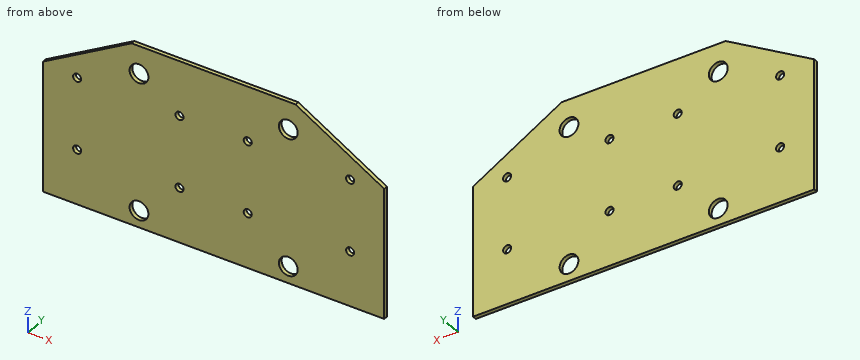
Autodesk Inventor part; units mm, degrees
ref_plane "YZ Plane" through (0, 0, 0) normal (1, 0, 0) x (0, 1, 0)
ref_plane "XZ Plane" through (0, 0, 0) normal (0, 1, 0) x (-1, 0, 0)
ref_plane "XY Plane" through (0, 0, 0) normal (0, 0, 1) x (1, 0, 0)
sketch "Sketch1" plane through (0, 0, 0) normal (0, 1, 0) x (-1, 0, 0)
  line L0 (-63.5, 33.655) -> (63.5, 33.655)
  line L1 (63.5, 33.655) -> (63.5, -33.655)
  line L2 (63.5, -33.655) -> (-63.5, -33.655)
  line L3 (-63.5, -33.655) -> (-63.5, 33.655)
  line L4 (-63.5, 33.655) -> (63.5, -33.655) construction
  line L5 (63.5, 33.655) -> (-63.5, -33.655) construction
  point P0 (0, 0)
  dimension "d0" = 127
  dimension "d1" = 67.31
extrude "Extrusion1" add sketch "Sketch1" along normal mid plane 1.524
sketch "Sketch2" plane through (0, 0.762, 0) normal (0, 1, 0) x (1, 0, 0)
  line L0 (63.5, 33.655) -> (-63.5, 33.655)
  line L1 (-63.5, -33.655) -> (63.5, -33.655)
  line L2 (-63.5, 33.655) -> (-63.5, -33.655)
  line L3 (63.5, -33.655) -> (63.5, 33.655)
  point P0 (0, 0)
  point P1 (-50.8, 13.335)
  point P2 (-12.7, 13.335)
  point P3 (12.7, 13.335)
  point P4 (50.8, 13.335)
  point P5 (50.8, -13.335)
  point P6 (12.7, -13.335)
  point P7 (-12.7, -13.335)
  point P8 (-50.8, -13.335)
  point P9 (-50.8, -33.655)
  point P10 (50.8, -33.655)
  point P11 (-63.5, -20.955)
  point P12 (63.5, -20.955)
  dimension "d5" = 20.32
  dimension "d6" = 20.32
  dimension "d7" = 12.7
  dimension "d8" = 50.8
  dimension "d9" = 12.7
  dimension "d10" = 50.8
hole "Hole1" at (-50.8, 0.762, -13.335) at (-12.7, 0.762, -13.335) at (12.7, 0.762, -13.335) at (50.8, 0.762, -13.335) at (50.8, 0.762, 13.335) at (12.7, 0.762, 13.335) at (-12.7, 0.762, 13.335) at (-50.8, 0.762, 13.335) direction (0, -1, 0) diameter 3 depth 25.4 tip angle 118
chamfer "Chamfer1" distance 19.05 angle 60 1 edges at (-63.5, 0, 33.655) measured on face at (-63.5, -0.254, 11.2183)
sketch "Sketch4" plane through (0, -0.762, 0) normal (0, -1, 0) x (1, 0, 0)
  circle A0 centre (-27.7751, -27.4042) radius 1.7018
  circle A1 centre (-27.7751, 23.3958) radius 1.7018
  circle A2 centre (27.7749, 23.3958) radius 1.7018
  circle A3 centre (27.7749, -27.4042) radius 1.7018
  point P0 (0, 0)
hole "Hole3" at (-27.7751, -0.762, -27.4042) at (-27.7751, -0.762, 23.3958) at (27.7749, -0.762, 23.3958) at (27.7749, -0.762, -27.4042) direction (0, 1, 0) diameter 7 end through all
chamfer "Chamfer2" distance 19.05 angle 60 1 edges at (63.5, 0, 33.655) measured on face at (63.5, 0.254, 11.2183)
properties part number "DPLX_P023 Spark Gap Shielding Bottom" material "Polyethylene, High Density"
Can you work these out from the model? Positions are in its coordinate system, mm. Give positions to 0.01 mm unless a question says otherwise; leave off trailing zeros. Order: outer loops, then holes, each group sorted by start corner. A loop starts at its lowest first (then second) coordinate and runs counter-clockwise, first axis right, second up. Notation, with made-up numbers: M 39,3.25 L 98,3.25 A17 cw 98,8.25 Z; hole C 1,4.25 d3. An arc over 180 degrees is marked long. One line per item, written item: value.
Item 1: Please list where these lines run through material, in increasing order: line 1 (Z direction, x = -12.7, y = 0.2) (3 decimals); line 2 (X direction, y = 0.5, z = -24.5); line 3 (Z direction, x = -29.5, y = 0.65) (3 decimals).
Verdict:
line 1: -33.655 to -14.835, -11.835 to 11.835, 14.835 to 33.655
line 2: -63.5 to -29.73, -25.82 to 25.82, 29.73 to 63.5
line 3: -33.655 to -30.45, -24.359 to 20.35, 26.441 to 33.655
Item 2: If we section it at A-A on x = -12.7: Write out the boundary of the cut face in (y, z) (3 decimals), and give its area (3 significant figures).
Verdict:
outline: M -0.762,-33.655 L 0.762,-33.655 L 0.762,-14.835 L -0.762,-14.835 Z; M -0.762,-11.835 L 0.762,-11.835 L 0.762,11.835 L -0.762,11.835 Z; M -0.762,14.835 L 0.762,14.835 L 0.762,33.655 L -0.762,33.655 Z
area: 93.4 mm2
Item 3: If we section it at D-D on x = -32.5: Write out the boundary of the cut face in (y, z) (3 decimals).
Verdict:
outline: M -0.762,-33.655 L 0.762,-33.655 L 0.762,32.503 L -0.762,32.503 Z
Item 4: If we section it at B-B on y = 0.45: State how many separate pieces and enclosed holes the cut face has, and give its area (3 significant figures).
Verdict:
separate pieces: 1
enclosed holes: 12
area: 7,710 mm2
Item 5: If we section it at C-C on x = -50.8: Write out the boundary of the cut face in (y, z) (3 decimals).
Verdict:
outline: M -0.762,-33.655 L 0.762,-33.655 L 0.762,-14.835 L -0.762,-14.835 Z; M -0.762,-11.835 L 0.762,-11.835 L 0.762,11.835 L -0.762,11.835 Z; M -0.762,14.835 L 0.762,14.835 L 0.762,21.937 L -0.762,21.937 Z
